Part model, mm, in its own coordinate system. A direction names the side the tool comes from. Give positions to 0.01 mm unless a question says otherwise; leave off trailing zeros. Write each loop counter-clockwise with the first axis right and the second up, starting at its lowest first coordinate (ties: lowest second). Pieces come first, ordered by that corner, then holes. Notation, with made-up numbers: (56.5, 38) - (105.5, 38) arc R28 ccw to (105.5, 70) - close; hole circle Ø7 at (38, 75). An arc over 180 degrees is marked (long way). Answer in a Markdown table with one row per item. Add a question column.
1. Pull direction Z, two halves, no side cores. Call faces 1 (the flat face through (59, 176.549, -17)), 2 (the flat face through (1, 187, 13.5)), 3 (the flat face through (-1, 180, 21.5)): released by +Z, released by -Z, zero draft, split by the parting line, or undercut.
2. Which spindle directions (+Z, -Z, +X, -X, +Y, -Y) get a long thin tool onto all of the face, cutting with end or side? Do faces 4 (the cylindrical face through (-1, 160, 0)), 5 (the flat face through (59, 176.549, 18)), 6 (the flat face through (-60, 176.549, 18)). Say none if no direction does.
3. Band-saw the part on D-D on x = 29. Write the cut outline in (y, z).
4. Drop flat-ended pins along their axis: pin 1 Ø5 at (x, z) = (-59.5, -15.5) entering from -Y; pin 2 Ø3 at (y, z) = (202.5, -12.5) entering from -X; pin 3 Ø6.5 at (x, z) = (-59, 17) entering from -Y; pin 4 Ø12 at (x, y) = (-28.5, 198.55) entering from +Z. Give the stop position or say it passes through.
5. Band-saw the part on A-A on x = -28.5. Write the cut outline in (y, z).
6. Band-saw the part on C-C on y = 204. Write the cut outline in (x, z).
7. Band-saw the part on B-B on z = 15. Write the cut outline in (x, y), plus the area to 3 significant figures.
8. Probe line 1 along Z through (x, y) = (-54, 182); line 2 along X through (y, z) = (168, -14); line 3 along Y through (x, z) = (-28, 16). List the from-to ranges inside material, lowest first.
```python
from build123d import *

# Parameters (mm, degrees)
SKETCH2_R           = 7.5
BOSS_EXTRUDE1_DEPTH = 21.5
SKETCH1_W           = 13.5
SKETCH1_H           = 90
CUT_EXTRUDE2_DEPTH  = 63


with BuildPart() as part:
    # Sketch2 → Boss-Extrude1 (new, symmetric)
    with BuildSketch(Plane.XY):
        with BuildLine():
            Line((-56.5, 158.548888359), (56.5, 158.548888359))
            Line((56.5, 158.548888359), (56.5, 176.548888359))
            Line((56.5, 176.548888359), (62.5, 176.548888359))
            Line((62.5, 176.548888359), (62.5, 183.691023983))
            ThreePointArc((62.5, 183.691023983), (61.503173004, 186.686788643), (58.91015764, 188.488049669))
            Line((58.91015764, 188.488049669), (-24.26952708, 212.939965417))
            ThreePointArc((-24.26952708, 212.939965417), (-32.207333005, 213.083525678), (-39.106601718, 209.155490077))
            Line((-39.106601718, 209.155490077), (-61.035533906, 187.226557889))
            ThreePointArc((-61.035533906, 187.226557889), (-62.119397663, 185.604441145), (-62.5, 183.691023983))
            Line((-62.5, 183.691023983), (-62.5, 176.548888359))
            Line((-62.5, 176.548888359), (-56.5, 176.548888359))
            Line((-56.5, 176.548888359), (-56.5, 158.548888359))
        make_face()
        with Locations((-28.5, 198.548888359)):
            Circle(SKETCH2_R, mode=Mode.SUBTRACT)
    extrude(amount=BOSS_EXTRUDE1_DEPTH, both=True)

    # Sketch1 → Cut-Extrude2 (cut, symmetric)
    with BuildSketch(Plane(origin=(0, 0, 0), x_dir=(0, 0, -1), z_dir=(1, 0, 0))):
        with BuildLine():
            ThreePointArc((21.5, 158.548888359), (10.774457353, 159.63680988), (0, 160))
            ThreePointArc((0, 160), (-10.774457353, 159.63680988), (-21.5, 158.548888359))
            Line((-21.5, 158.548888359), (21.5, 158.548888359))
        make_face()
        with BuildLine():
            ThreePointArc((160, 0), (120.498962651, 105.261578936), (21.5, 158.548888359))
            Line((21.5, 158.548888359), (-21.5, 158.548888359))
            ThreePointArc((-21.5, 158.548888359), (-105.261578936, -120.498962651), (160, 0))
        make_face()
        with Locations((6.75, 215)):
            Rectangle(SKETCH1_W, SKETCH1_H)
        with Locations((-6.75, 215)):
            Rectangle(SKETCH1_W, SKETCH1_H)
    extrude(amount=CUT_EXTRUDE2_DEPTH, both=True, mode=Mode.SUBTRACT)


solid = part.part
```
Values:
| question | item | result |
|---|---|---|
| 1 | face 1 | zero draft |
| 1 | face 2 | undercut |
| 1 | face 3 | released by +Z |
| 2 | face 4 | +X, -X, -Y |
| 2 | face 5 | +Z, -Z, +X, -Y |
| 2 | face 6 | +Z, -Z, -X, -Y |
| 3 | outline | (158.55, -21.5) - (197.28, -21.5) - (197.28, -13.5) - (170, -13.5) - (170, 13.5) - (197.28, 13.5) - (197.28, 21.5) - (158.55, 21.5) arc R160 cw to start |
| 4 | pin 1 | stops at y = 176.55 |
| 4 | pin 2 | stops at x = -46.88 |
| 4 | pin 3 | stops at y = 158.86 |
| 4 | pin 4 | passes through |
| 5 | outline | (158.55, -21.5) - (191.05, -21.5) - (191.05, -13.5) - (170, -13.5) - (170, 13.5) - (191.05, 13.5) - (191.05, 21.5) - (158.55, 21.5) arc R160 cw to start; (206.05, -21.5) - (213.55, -21.5) - (213.55, -13.5) - (206.05, -13.5) - close; (206.05, 13.5) - (213.55, 13.5) - (213.55, 21.5) - (206.05, 21.5) - close |
| 6 | outline | (-44.26, -21.5) - (-33.65, -21.5) - (-33.65, -13.5) - (-44.26, -13.5) - close; (-44.26, 13.5) - (-33.65, 13.5) - (-33.65, 21.5) - (-44.26, 21.5) - close; (-23.35, -21.5) - (6.14, -21.5) - (6.14, -13.5) - (-23.35, -13.5) - close; (-23.35, 13.5) - (6.14, 13.5) - (6.14, 21.5) - (-23.35, 21.5) - close |
| 7 | outline | (-62.5, 176.55) - (-56.5, 176.55) - (-56.5, 159.3) - (56.5, 159.3) - (56.5, 176.55) - (62.5, 176.55) - (62.5, 183.69) arc R5 ccw to (58.91, 188.49) - (-24.27, 212.94) arc R15 ccw to (-39.11, 209.16) - (-61.04, 187.23) arc R5 ccw to (-62.5, 183.69) - close; hole circle Ø15 at (-28.5, 198.55) |
| 7 | area | 4,840 mm² |
| 8 | line 1 | z = -21.5 to -13.5, 13.5 to 21.5 |
| 8 | line 2 | x = -56.5 to 56.5 |
| 8 | line 3 | y = 159.2 to 191.07, 206.03 to 213.54 |
